Work out the finished part from the listing and answer in its coordinate system (mm). Face numbers are marked on the shaded views. A direction names the side the tool comes from. Coordinates: 2 decimals unless noted, no trailing zeros. Order: outer loops, then holes, each group sorted by start corner. A loop starts at its lowest first (then second) coordinate and runs counter-clockwise, first axis right, second up.
1. A tool of negligible diameter and unlimited length cuts with its end or side. For the marked faces 5 and 6, from which of +Z, -Z, +X, -X, +Y, -Y can it reach the whole face along a straight path? Write none if from no direction.
2. The part is cut by section A-A, the plane y = 3. Count the separate pieces of the cut face and the enclosed holes in it, then the cut area to 3 significant figures.
3. The part is cut by section B-B, the plane y = 13.5. Give the vertices of the cut face in (x, z), then the cut area to 3 significant figures.
4. Find the intervals of material crossed by probe 1 along X at (y, z) = (14.5, -38); probe 2 along X at (y, z) = (42.5, 3); probe 3 along Z at (x, y) = (0.25, 3.25), in increasing order.
5. The part is cut by section D-D, the plane z = 6. Give the vertices of the cut face in (x, y).
6. The part is cut by section C-C, the plane x = 0.25. Give the vertices of the cut face in (y, z).
7. Flat-ended cylindrical pins translate along their axes: pin 1 Ø5 at (x, z) = (-44, 37.5) entering from +Y; pin 2 Ø4 at (x, z) = (0, 38.5) entering from +Y; pin 3 Ø6.5 at (x, z) = (49.5, 32) entering from +Y. Find the tip coordinate at first contact, or state that the pin passes through.
8. Determine the mould class of the marked faces 1, 2, 3 and 4 for opening direction Z: +Z half, -Z half, draft (parallel to the pull), parting line (faces both ways), or undercut.
```python
from build123d import *

# Parameters (mm, degrees)
SKETCH1_W             = 173
SKETCH1_H             = 103
SKETCH1_W_2           = 165
SKETCH1_H_2           = 95
BOSS_EXTRUDE1_DEPTH   = 45
SKETCH1_3_W           = 173
SKETCH1_3_H           = 103
BOSS_EXTRUDE2_DEPTH   = 4
SKETCH5_W             = 6
SKETCH5_H             = 95
BOSS_EXTRUDE3_DEPTH   = 32
SKETCH6_R             = 5
SKETCH6_R_2           = 2.5
STANDOFFINSERTS_DEPTH = 10
SKETCH7_W             = 25.4
SKETCH7_H             = 3.5
CUT_EXTRUDE1_DEPTH    = 104
SKETCH8_W             = 8
SKETCH8_H             = 25
BOSS_EXTRUDE5_DEPTH   = 25
SKETCH9_R             = 10.16
CUT_EXTRUDE2_DEPTH    = 10


with BuildPart() as part:
    # Sketch1 → Boss-Extrude1 (new body)
    with BuildSketch(Plane(origin=(0, 0, 0), x_dir=(1, 0, 0), z_dir=(0, 1, 0))):
        Rectangle(SKETCH1_W, SKETCH1_H)
        Rectangle(SKETCH1_W_2, SKETCH1_H_2, mode=Mode.SUBTRACT)
    extrude(amount=BOSS_EXTRUDE1_DEPTH)

    # Sketch1_3 → Boss-Extrude2 (add)
    with BuildSketch(Plane(origin=(0, 0, 0), x_dir=(1, 0, 0), z_dir=(0, 1, 0))):
        Rectangle(SKETCH1_3_W, SKETCH1_3_H)
    extrude(amount=-BOSS_EXTRUDE2_DEPTH)

    # Sketch5 → Boss-Extrude3 (add)
    with BuildSketch(Plane(origin=(0, 0, 0), x_dir=(1, 0, 0), z_dir=(0, 1, 0))):
        with Locations((11, 0)):
            Rectangle(SKETCH5_W, SKETCH5_H)
    extrude(amount=BOSS_EXTRUDE3_DEPTH)

    # Sketch6 → StandoffInserts (add)
    with BuildSketch(Plane(origin=(0, 0, 0), x_dir=(1, 0, 0), z_dir=(0, 1, 0))):
        with Locations((-74.75, -38)):
            Circle(SKETCH6_R)
        with Locations((-74.75, -38)):
            Circle(SKETCH6_R_2, mode=Mode.SUBTRACT)
        with Locations((0.25, -38)):
            Circle(SKETCH6_R)
        with Locations((0.25, -38)):
            Circle(SKETCH6_R_2, mode=Mode.SUBTRACT)
        with Locations((-74.75, 38)):
            Circle(SKETCH6_R)
        with Locations((-74.75, 38)):
            Circle(SKETCH6_R_2, mode=Mode.SUBTRACT)
        with Locations((0.25, 38)):
            Circle(SKETCH6_R)
        with Locations((0.25, 38)):
            Circle(SKETCH6_R_2, mode=Mode.SUBTRACT)
    extrude(amount=STANDOFFINSERTS_DEPTH)

    # Sketch7 → Cut-Extrude1 (cut, through all)
    with BuildSketch(Plane(origin=(0, 0, -51.5), x_dir=(-1, 0, 0), z_dir=(0, 0, -1))):
        with Locations((51.5, 31)):
            Rectangle(SKETCH7_W, SKETCH7_H)
    extrude(amount=-CUT_EXTRUDE1_DEPTH, mode=Mode.SUBTRACT)

    # Sketch8 → Boss-Extrude5 (add)
    with BuildSketch(Plane(origin=(0, 0, 0), x_dir=(1, 0, 0), z_dir=(0, 1, 0))):
        with Locations((49.90120524, -35)):
            Rectangle(SKETCH8_W, SKETCH8_H)
    extrude(amount=BOSS_EXTRUDE5_DEPTH)

    # Sketch9 → Cut-Extrude2 (cut)
    with BuildSketch(Plane.ZY.offset(86.5)):
        with Locations((0, 31)):
            Circle(SKETCH9_R)
    extrude(amount=-CUT_EXTRUDE2_DEPTH, mode=Mode.SUBTRACT)


solid = part.part
```
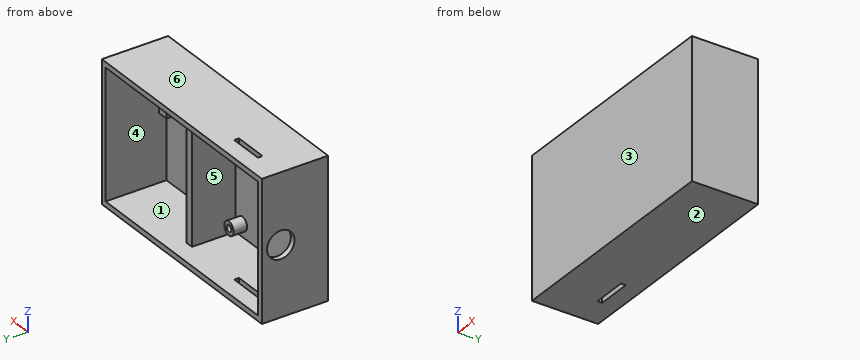
Geometry says:
1. face 5: +Y
1. face 6: +Z, +X, -X, +Y, -Y
2. separate pieces: 5
2. enclosed holes: 6
2. area: 3,150 mm2
3. outline: (-86.5, -51.5) - (86.5, -51.5) - (86.5, 51.5) - (-86.5, 51.5) - close; hole (-82.5, -47.5) - (8, -47.5) - (8, 47.5) - (-82.5, 47.5) - close; hole (14, -47.5) - (82.5, -47.5) - (82.5, 47.5) - (53.9, 47.5) - (53.9, 22.5) - (45.9, 22.5) - (45.9, 47.5) - (14, 47.5) - close
3. area: 2,910 mm2
4. probe 1: x = -86.5 to -82.5, 8 to 14, 82.5 to 86.5
4. probe 2: x = -86.5 to -82.5, 82.5 to 86.5
4. probe 3: z = -51.5 to -47.5, -43 to -40.5, -35.5 to -33, 33 to 35.5, 40.5 to 43, 47.5 to 51.5
5. outline: (-86.5, -4) - (86.5, -4) - (86.5, 45) - (82.5, 45) - (82.5, 0) - (14, 0) - (14, 32) - (8, 32) - (8, 0) - (-82.5, 0) - (-82.5, 22.8) - (-86.5, 22.8) - close; (-86.5, 39.2) - (-82.5, 39.2) - (-82.5, 45) - (-86.5, 45) - close
6. outline: (-4, -51.5) - (45, -51.5) - (45, -47.5) - (0, -47.5) - (0, -43) - (10, -43) - (10, -40.5) - (0, -40.5) - (0, -35.5) - (10, -35.5) - (10, -33) - (0, -33) - (0, 33) - (10, 33) - (10, 35.5) - (0, 35.5) - (0, 40.5) - (10, 40.5) - (10, 43) - (0, 43) - (0, 47.5) - (45, 47.5) - (45, 51.5) - (-4, 51.5) - close
7. pin 1: stops at y = 0
7. pin 2: stops at y = 10
7. pin 3: stops at y = 25
8. face 1: undercut
8. face 2: -Z half
8. face 3: draft
8. face 4: undercut
